from build123d import *

# Parameters (mm, degrees)
F0_W      = 127
F0_H      = 127
F1_DEPTH  = 6.35
F3_DEPTH  = 6.35
F5_DEPTH  = 5.08
F6_W      = 43.18
F6_H      = 43.18
F7_DEPTH  = 6.35
F9_DEPTH  = 6.35
F11_DEPTH = 5.08
F12_W     = 38.1
F12_H     = 38.1
F13_DEPTH = 6.35
F14_R     = 3.4925
F15_DEPTH = 2.54
F17_DEPTH = 6.35


with BuildPart() as f1:
    # F0 (on Top) → F1 (new body)
    with BuildSketch(Plane.XY):
        with Locations((0.5442854017, -13.0122138653)):
            Rectangle(F0_W, F0_H)
    extrude(amount=F1_DEPTH)

    # F2 (on face) → F3 (join)
    with BuildSketch(Plane.XY.offset(6.35)):
        Polygon((-53.7375879309, -17.5850009601), (-58.7414534923, -22.4585576124), (-9.1197857594, -73.4070069648), (-4.115920198, -68.5334503124), align=None)
    extrude(amount=F3_DEPTH)

    # F4 (on face) → F5 (cut)
    with BuildSketch(Plane.XY.offset(12.7)):
        Polygon((-22.838354329, -49.3104166932), (-27.8422198903, -54.1839733455), (-18.1633084233, -64.1216790535), (-13.1594428619, -59.2481224011), align=None)
    extrude(amount=-F5_DEPTH, mode=Mode.SUBTRACT)

    # F6 (on face) → F7 (join)
    with BuildSketch(Plane.XY.offset(6.35)):
        with Locations((35.4591379873, -45.8693522716)):
            Rectangle(F6_W, F6_H)
    extrude(amount=F7_DEPTH)

    # F8 (on face) → F9 (join)
    with BuildSketch(Plane.XY.offset(6.35)):
        Polygon((34.285597458, 39.0348099981), (-31.2195517093, -24.764477087), (-26.345995057, -29.7683426483), (39.1591541104, 34.0309444367), align=None)
    extrude(amount=F9_DEPTH)

    # F10 (on face) → F11 (cut)
    with BuildSketch(Plane.XY.offset(12.7)):
        Polygon((-11.3444998697, -5.4070043651), (-23.882560582, -17.618553305), (-19.0090039296, -22.6224188664), (-6.4709432174, -10.4108699265), align=None)
        Polygon((28.5604737616, 33.4587779618), (18.924622147, 24.0738598097), (23.7981787993, 19.0699942484), (33.434030414, 28.4549124004), align=None)
    extrude(amount=-F11_DEPTH, mode=Mode.SUBTRACT)

    # F12 (on face) → F13 (join)
    with BuildSketch(Plane.XY.offset(6.35)):
        with Locations((-39.4052062184, 28.9046873478)):
            Rectangle(F12_W, F12_H)
    extrude(amount=F13_DEPTH)

    # F14 (on face) → F15 (cut)
    with BuildSketch(Plane.XY.offset(6.35)):
        with Locations((-41.9958606362, -9.7006224096)):
            Circle(F14_R)
    extrude(amount=-F15_DEPTH, mode=Mode.SUBTRACT)

    # F16 (on face) → F17 (join)
    with BuildSketch(Plane.XY.offset(6.35)):
        Polygon((-43.8297687504, -15.1278137338), (-47.9132530889, -12.1059673352), (-49.6608870253, -18.737553844), align=None)
    extrude(amount=F17_DEPTH)


solid = f1.part
Check sheet for the modelled part. Datum: model origin and axes. Units: mm. A direction names the side the tool comes from. Round coordinates to 2 decimals unless told otherwise and drop trailing zeros. Loops run counter-clockwise (first coordinate to the right, second up) from the corner with the lowest first, then second, coordinate; pieces in that order, holes last. Notation, with made-up numbers: (23, 84) - (64, 84) arc R14 ccw to (64, 99) - close; hole circle Ø3 at (-5, -7). An arc over 180 degrees is marked (long way). Answer as CSV lines item,"result". Start each with the question number.
Item 1: Section check C-C (y = -62). Record the boundary of the cut face in (x, z).
Item 2: Scan lines: line 1 (Y direction, x = -30.5, z = 8); line 2 (X direction, y = -18, z = 11.25); line 3 (Y direction, x = 46, z = 7.75). Record each from-to range of solid material in increasing order. Write a range as [from, to].
Item 3: Section check A-A (z = 11.25). Count the separate pieces of the cut face and the enclosed holes in it, and give its area (3 significant figures).
Item 4: Section check D-D (x = 9). Record the boundary of the cut face in (y, z), and give its area (3 significant figures).
Item 5: Depth check by flat-ended pin: P1, Ø5, axis at x = -35.5, z = 9.5, coming from the -Y side; P2, Ø1, axis at y = -4.5, z = 9.5, coming from the +X side; P3, Ø3, axis at y = -57.5, z = 10.5, coming from the -X side. Enter the tip coordinate at first touch or a pass-through.
Item 6: Set-up check for faces 1 (the cylindrical face through (-44.57, -7.34, 5.1)), 2 (the flat face through (13.869, -46, 9)), 3 (the flat face through (-34.278, -47.576, 9.481)): record each of +Z, -Z, +X, -X, +Y, -Y from which the full face is reachable in a straight line by a thin tool's end or side.
Item 7: Section check B-B (x = 47). Record the boundary of the cut face in (y, z), and give its area (3 significant figures).
Item 8: Release check for a two-part mould opening along Y. For faces 4 (the flat face through (-41, -36, 12.7)), 5 (the flat face through (35, -24.279, 9)), 6 (the flat face through (0, -76.512, 3)), 7 (the flat face through (-15.7, -61.72, 10.2)) record: +Y half, -Y half, draft (parallel to the pull), parting line (faces both ways), or undercut.
Report:
1,outline,"(-62.96, 0) - (64.04, 0) - (64.04, 6.35) - (57.05, 6.35) - (57.05, 12.7) - (13.87, 12.7) - (13.87, 6.35) - (-10.48, 6.35) - (-10.48, 12.7) - (-15.98, 12.7) - (-15.98, 7.62) - (-20.23, 7.62) - (-20.23, 6.35) - (-62.96, 6.35) - close"
2,line 1,"y = [-51.46, -41.44], [-25.5, -24.06], [9.85, 47.95]"
2,line 2,"x = [-54.16, -53.33], [-49.47, -48.47], [-24.27, -23.51]"
2,line 3,"y = [-67.46, -24.28]"
3,separate pieces,"8"
3,enclosed holes,"0"
3,area,"4,150 mm2"
4,outline,"(-76.51, 0) - (50.49, 0) - (50.49, 6.35) - (14.41, 6.35) - (14.41, 12.7) - (4.66, 12.7) - (4.66, 6.35) - (-76.51, 6.35) - close"
4,area,"868 mm2"
5,P1,"stops at y = -48.89"
5,P2,"stops at x = 0.11"
5,P3,"stops at x = 13.87"
6,face 1,"+Z"
6,face 2,"+Z, -Y"
6,face 3,"+Z, -X, -Y"
7,outline,"(-76.51, 0) - (50.49, 0) - (50.49, 6.35) - (-24.28, 6.35) - (-24.28, 12.7) - (-67.46, 12.7) - (-67.46, 6.35) - (-76.51, 6.35) - close"
7,area,"1,080 mm2"
8,face 4,"draft"
8,face 5,"undercut"
8,face 6,"-Y half"
8,face 7,"+Y half"
